from build123d import *

# Parameters (mm, degrees)
SKETCH1_W               = 170
SKETCH1_H               = 80
BOSS_EXTRUDE1_DEPTH     = 7
SKETCH2_W               = 7
SKETCH2_H               = 18
BOSS_EXTRUDE2_DEPTH     = 18
SKETCH3_R               = 2
CUT_EXTRUDE1_DEPTH      = 20
SKETCH4_W               = 7
SKETCH4_H               = 8
CUT_EXTRUDE2_DEPTH      = 2.3
SKETCH6_W               = 20
SKETCH6_H               = 19
CUT_EXTRUDE4_DEPTH      = 11
SKETCH7_R               = 2
CUT_EXTRUDE5_DEPTH      = 25
SKETCH7_2_R             = 2
CUT_EXTRUDE6_DEPTH      = 25
SKETCH8_W               = 170
SKETCH8_H               = 80
BOSS_EXTRUDE3_DEPTH     = 20
SKETCH9_W               = 134
SKETCH9_H               = 80
CUT_EXTRUDE7_DEPTH      = 20
SKETCH12_W              = 134
SKETCH12_H              = 28
BOSS_EXTRUDE4_DEPTH     = 20
SKETCH10_R              = 2
CUT_EXTRUDE9_DEPTH      = 1
CUT_EXTRUDE9_DEPTH_BACK = 46
SKETCH13_W              = 112.5
SKETCH13_H              = 22
CUT_EXTRUDE10_DEPTH     = 20
SKETCH14_R              = 2
CUT_EXTRUDE11_DEPTH     = 10


with BuildPart() as part:
    # Sketch1 → Boss-Extrude1 (new body)
    with BuildSketch(Plane(origin=(0, 0, 0), x_dir=(1, 0, 0), z_dir=(0, 1, 0))):
        with Locations((5.170316302, -0.291970803)):
            Rectangle(SKETCH1_W, SKETCH1_H)
    extrude(amount=BOSS_EXTRUDE1_DEPTH)

    # Sketch2 → Boss-Extrude2 (add)
    with BuildSketch(Plane(origin=(0, 7, 0), x_dir=(1, 0, 0), z_dir=(0, 1, 0))):
        with Locations((-76.329683698, -0.291970803)):
            Rectangle(SKETCH2_W, SKETCH2_H)
    extrude(amount=BOSS_EXTRUDE2_DEPTH)

    # Sketch3 → Cut-Extrude1 (cut)
    with BuildSketch(Plane(origin=(0, 0, -8.708029197), x_dir=(-1, 0, 0), z_dir=(0, 0, -1))):
        with Locations((76.329683698, 17)):
            Circle(SKETCH3_R)
    extrude(amount=-CUT_EXTRUDE1_DEPTH, mode=Mode.SUBTRACT)

    # Sketch4 → Cut-Extrude2 (cut)
    with BuildSketch(Plane.XY.offset(9.291970803)):
        with Locations((-76.329683698, 17)):
            Rectangle(SKETCH4_W, SKETCH4_H)
    extrude(amount=-CUT_EXTRUDE2_DEPTH, mode=Mode.SUBTRACT)

    # Sketch6 → Cut-Extrude4 (cut)
    with BuildSketch(Plane(origin=(0, 7, 0), x_dir=(1, 0, 0), z_dir=(0, 1, 0))):
        with Locations((80.170316302, 17.208029197)):
            Rectangle(SKETCH6_W, SKETCH6_H)
    extrude(amount=-CUT_EXTRUDE4_DEPTH, mode=Mode.SUBTRACT)

    # Sketch7 → Cut-Extrude5 (cut)
    with BuildSketch(Plane.XY.offset(-26.708029197)):
        with Locations((80.170316302, 3.5)):
            Circle(SKETCH7_R)
    extrude(amount=-CUT_EXTRUDE5_DEPTH, mode=Mode.SUBTRACT)

    # Sketch7<2> → Cut-Extrude6 (cut)
    with BuildSketch(Plane.XY.offset(-26.708029197)):
        with Locations((80.170316302, 3.5)):
            Circle(SKETCH7_2_R)
    extrude(amount=CUT_EXTRUDE6_DEPTH, mode=Mode.SUBTRACT)

    # Sketch8 → Boss-Extrude3 (add)
    with BuildSketch(Plane.XZ):
        with Locations((5.170316302, 0.291970803)):
            Rectangle(SKETCH8_W, SKETCH8_H)
    extrude(amount=BOSS_EXTRUDE3_DEPTH)

    # Sketch9 → Cut-Extrude7 (cut)
    with BuildSketch(Plane(origin=(0, 7, 0), x_dir=(1, 0, 0), z_dir=(0, 1, 0))):
        with Locations((-5.829683698, -0.291970803)):
            Rectangle(SKETCH9_W, SKETCH9_H)
    extrude(amount=-CUT_EXTRUDE7_DEPTH, mode=Mode.SUBTRACT)

    # Sketch12 → Boss-Extrude4 (add)
    with BuildSketch(Plane(origin=(0, -13, 0), x_dir=(1, 0, 0), z_dir=(0, 1, 0))):
        with Locations((-5.829683698, -26.291970803)):
            Rectangle(SKETCH12_W, SKETCH12_H)
    extrude(amount=BOSS_EXTRUDE4_DEPTH)

    # Sketch10 → Cut-Extrude9 (cut, two sides)
    with BuildSketch(Plane.XZ.offset(20)) as cut_extrude9_sk:
        with Locations((83.670316302, 28.191970803)):
            Circle(SKETCH10_R)
        with Locations((-58.329683698, 28.191970803)):
            Circle(SKETCH10_R)
    extrude(amount=CUT_EXTRUDE9_DEPTH, mode=Mode.SUBTRACT)
    extrude(cut_extrude9_sk.sketch, amount=-CUT_EXTRUDE9_DEPTH_BACK, mode=Mode.SUBTRACT)

    # Sketch13 → Cut-Extrude10 (cut)
    with BuildSketch(Plane(origin=(0, 7, 0), x_dir=(1, 0, 0), z_dir=(0, 1, 0))):
        with Locations((4.920316302, -23.291970803)):
            Rectangle(SKETCH13_W, SKETCH13_H)
    extrude(amount=-CUT_EXTRUDE10_DEPTH, mode=Mode.SUBTRACT)

    # Sketch14 → Cut-Extrude11 (cut)
    with BuildSketch(Plane(origin=(0, -13, 0), x_dir=(1, 0, 0), z_dir=(0, 1, 0))):
        with Locations((-39.829683698, 24.708029197)):
            Circle(SKETCH14_R)
        with Locations((-39.829683698, 9.708029197)):
            Circle(SKETCH14_R)
        with Locations((-14.829683698, 9.708029197)):
            Circle(SKETCH14_R)
        with Locations((-14.829683698, 24.708029197)):
            Circle(SKETCH14_R)
    extrude(amount=-CUT_EXTRUDE11_DEPTH, mode=Mode.SUBTRACT)


with BuildPart() as body_2:
    # Mirror2: mirrored copy
    add(part.part.mirror(Plane(origin=(90.170316302, 7, -39.708029197), x_dir=(0, 0, 1), z_dir=(-1, 0, 0))))


solid = body_2.part
Design review of the part built by this model. Coordinates are the model's own, in mm. A direction names the side the tool comes from. Coordinates: 2 decimals unless noted, no trailing zeros. Loops run counter-clockwise (first coordinate to the right, second up) from the corner with the lowest first, then second, coordinate; pieces in that order, holes last. Notation, with made-up numbers: (-13.5, 4) -> (41.5, 4) arc R3 ccw to (41.5, 9) -> close; hole circle Ø3 at (-40, 76.5). An arc over 180 degrees is marked (long way). Use a Markdown table: item, result. Add a question column.
Item 1: We need section B-B, the plane x = 250.5. Write out the cut boundary in (y, z).
Item 2: Machinability: for faces 4 (the flat face through (100, 0, -17)), 5 (the flat face through (100, 4, -1.708)), 6 (the flat face through (119.17, -3, -2)), which of the approach directions +Z, -Z, +X, -X, +Y, -Y give a long, thin tool a straight path to every point of the face, cutting with its end or side? Answer none if there is none.
Item 3: Clearance check with flat-ended pins moving along their axes: P1, Ø5.5, axis at x = 258, y = 14.5, coming from the -Z side; P2, Ø2.5, axis at x = 100.17, y = 3.5, coming from the -Z side; P3, Ø5, axis at x = 238.67, z = 28.19, coming from the -Y side; P4, Ø5, axis at x = 162, z = -22, coming from the +Y side. State where each tip first meets the part, or that it passes through.
Item 4: We need section A-A, the plane y = 17. Write out the cut boundary in (x, z), and give its area (3 significant figures).
Item 5: We need section D-D, the plane y = -8.5. Write out the cut boundary in (x, z).
Item 6: Wall thickness on L1, parallel to X at y = -14.5, z = -8; L2, parallel to X at y = 3, z = -3; L3, parallel to X at y = 0.5, z = -25.5: over which ranges is each line inside the solid? List them lowest first. Write a range as from..to.
Item 7: We need section C-C, the plane y = 3.5. Write out the cut boundary in (x, z).
Item 8: The part is to be moulded in two halves that separate along Z. For faces 1 (the cylindrical face through (193.263, -16.451, -25.309)), 2 (the flat face through (257, 14, -8.708)), 3 (the flat face through (187, -13, -3)), say which applies: +Z half, -Z half, draft (parallel to the pull), parting line (faces both ways), or undercut.
Numbers:
| question | item | result |
|---|---|---|
| 1 | outline | (-20, -39.71) -> (-13, -39.71) -> (-13, 12.29) -> (7, 12.29) -> (7, 40.29) -> (-20, 40.29) -> close |
| 2 | face 4 | -X, +Y |
| 2 | face 5 | -Z |
| 2 | face 6 | -Z, +Y |
| 3 | P1 | stops at z = -8.71 |
| 3 | P2 | stops at z = -1.71 |
| 3 | P3 | stops at y = -20 |
| 3 | P4 | stops at y = -13 |
| 4 | outline | (253.17, -8.71) -> (254.67, -8.71) -> (254.67, 6.99) -> (253.17, 6.99) -> close; (258.67, -8.71) -> (260.17, -8.71) -> (260.17, 6.99) -> (258.67, 6.99) -> close |
| 4 | area | 47.1 mm^2 |
| 5 | outline | (90.17, -39.71) -> (119.17, -39.71) -> (119.17, 34.29) -> (231.67, 34.29) -> (231.67, 12.29) -> (253.17, 12.29) -> (253.17, -39.71) -> (260.17, -39.71) -> (260.17, 40.29) -> (90.17, 40.29) -> close; hole circle Ø4 at (96.67, 28.19); hole circle Ø4 at (238.67, 28.19) |
| 6 | L1 | x = 90.17..194.13, 196.21..219.13, 221.21..260.17 |
| 6 | L2 | x = 90.17..98.23, 102.11..119.17, 253.17..260.17 |
| 6 | L3 | x = 110.17..119.17, 253.17..260.17 |
| 7 | outline | (90.17, -39.71) -> (98.17, -39.71) -> (98.17, -26.71) -> (90.17, -26.71) -> close; (90.17, -7.71) -> (98.17, -7.71) -> (98.17, -1.71) -> (102.17, -1.71) -> (102.17, -7.71) -> (110.17, -7.71) -> (110.17, -26.71) -> (102.17, -26.71) -> (102.17, -39.71) -> (119.17, -39.71) -> (119.17, 34.29) -> (231.67, 34.29) -> (231.67, 12.29) -> (253.17, 12.29) -> (253.17, -39.71) -> (260.17, -39.71) -> (260.17, 40.29) -> (90.17, 40.29) -> close; hole circle Ø4 at (96.67, 28.19); hole circle Ø4 at (238.67, 28.19) |
| 8 | face 1 | undercut |
| 8 | face 2 | -Z half |
| 8 | face 3 | draft |
